from build123d import *

# Parameters (mm, degrees)
SKETCH1_R                = 103.1875
BASE_FLANGE1_DEPTH       = 4.7752
SKETCH6_R                = 4.9609375
CUT_EXTRUDE1_DEPTH       = 147.007269845
SKETCH7_R                = 38.1
CUT_EXTRUDE2_DEPTH       = 147.007269845
CUT_EXTRUDE6_DEPTH       = 147.007269845
FILLET2_R                = 1.5875
FILLET3_R                = 8.466666667
CIRPATTERN3_COUNT        = 14
FILLET2_OF_CIRPATTERN3_R = 1.5875
FILLET3_OF_CIRPATTERN3_R = 8.466666667


# Sheet-metal steps are written as plain solids
with BuildPart() as part:
    # Sketch1 → Base-Flange1 (new body)
    with BuildSketch(Plane.XY):
        Circle(SKETCH1_R)
    extrude(amount=-BASE_FLANGE1_DEPTH)

    # Sketch6 → Cut-Extrude1 (cut, through all)
    with BuildSketch(Plane.XY):
        with Locations((0, 47.534367171)):
            Circle(SKETCH6_R)
        with Locations((45.207869646, 14.688927273)):
            Circle(SKETCH6_R)
        with Locations((27.94, -38.456110858)):
            Circle(SKETCH6_R)
        with Locations((-27.94, -38.456110858)):
            Circle(SKETCH6_R)
        with Locations((-45.207869646, 14.688927273)):
            Circle(SKETCH6_R)
    extrude(amount=-CUT_EXTRUDE1_DEPTH, mode=Mode.SUBTRACT)

    # Sketch7 → Cut-Extrude2 (cut, through all)
    with BuildSketch(Plane.XY):
        Circle(SKETCH7_R)
    extrude(amount=-CUT_EXTRUDE2_DEPTH, mode=Mode.SUBTRACT)

    # Sketch14 → Cut-Extrude6 (cut, through all)
    with BuildSketch(Plane.XY):
        with BuildLine():
            ThreePointArc((0, 96.8375), (16.707624198, 79.710005113), (29.767032143, 59.661372951))
            ThreePointArc((29.767032143, 59.661372951), (25.116422432, 61.763427279), (20.318653947, 63.50360562))
            ThreePointArc((20.318653947, 63.50360562), (6.935369559, 81.376622779), (-9.620686715, 96.358413195))
            ThreePointArc((-9.620686715, 96.358413195), (-4.816304004, 96.717654138), (0, 96.8375))
        make_face()
    cut_extrude6 = extrude(amount=-CUT_EXTRUDE6_DEPTH, mode=Mode.SUBTRACT)

    # Fillet2
    fillet2_edges = [part.edges().sort_by_distance(p)[0] for p in [
        (-9.620686715, 96.358413195, -2.3876),
        (29.767032143, 59.661372951, -2.3876),
    ]]
    fillet(fillet2_edges, radius=FILLET2_R)

    # Fillet3
    fillet3_edges = [part.edges().sort_by_distance(p)[0] for p in [
        (0, 96.8375, -2.3876),
        (20.318653947, 63.50360562, -2.3876),
    ]]
    fillet(fillet3_edges, radius=FILLET3_R)

    # CirPattern3: Cut-Extrude6 ×14 about axis
    cirpattern3_axis = Axis((0, 0, 0), (0, 0, 1))
    for i in range(1, CIRPATTERN3_COUNT):
        add(cut_extrude6.rotate(cirpattern3_axis, i * 360 / CIRPATTERN3_COUNT), mode=Mode.SUBTRACT)

    # Fillet2 of CirPattern3
    fillet2_of_cirpattern3_edges = [part.edges().sort_by_distance(p)[0] for p in [
        (-50.47628783, 82.641670924, -2.3876),
        (0.933069674, 66.668470854, -2.3876),
        (-81.33444109, 52.556732194, -2.3876),
        (-28.085698687, 60.471060469, -2.3876),
        (-96.08331079, 12.062288086, -2.3876),
        (-51.541749975, 42.296614929, -2.3876),
        (-91.801702404, -30.821240111, -2.3876),
        (-64.789325562, 15.744806069, -2.3876),
        (-69.337640983, -67.600243707, -2.3876),
        (-65.204580633, -13.92545473, -2.3876),
        (-33.140409395, -90.990189973, -2.3876),
        (-52.705268828, -40.837608436, -2.3876),
        (9.620686715, -96.358413195, -2.3876),
        (-29.767032143, -59.661372951, -2.3876),
        (50.47628783, -82.641670924, -2.3876),
        (-0.933069674, -66.668470854, -2.3876),
        (81.33444109, -52.556732194, -2.3876),
        (28.085698687, -60.471060469, -2.3876),
        (96.08331079, -12.062288086, -2.3876),
        (51.541749975, -42.296614929, -2.3876),
        (91.801702404, 30.821240111, -2.3876),
        (64.789325562, -15.744806069, -2.3876),
        (69.337640983, 67.600243707, -2.3876),
        (65.204580633, 13.92545473, -2.3876),
        (33.140409395, 90.990189973, -2.3876),
        (52.705268828, 40.837608436, -2.3876),
    ]]
    fillet(fillet2_of_cirpattern3_edges, radius=FILLET2_OF_CIRPATTERN3_R)

    # Fillet3 of CirPattern3
    fillet3_of_cirpattern3_edges = [part.edges().sort_by_distance(p)[0] for p in [
        (-42.016216587, 87.247572746, -2.3876),
        (-9.24670721, 66.030705212, -2.3876),
        (-75.710606183, 60.377193687, -2.3876),
        (-36.980644601, 55.479613823, -2.3876),
        (-94.409581696, 21.548370942, -2.3876),
        (-57.39011179, 33.940104503, -2.3876),
        (-94.409581696, -21.548370942, -2.3876),
        (-66.432763496, 5.678341239, -2.3876),
        (-75.710606183, -60.377193687, -2.3876),
        (-62.317591648, -23.708087148, -2.3876),
        (-42.016216587, -87.247572746, -2.3876),
        (-45.859656498, -48.398838115, -2.3876),
        (0, -96.8375, -2.3876),
        (-20.318653947, -63.50360562, -2.3876),
        (42.016216587, -87.247572746, -2.3876),
        (9.24670721, -66.030705212, -2.3876),
        (75.710606183, -60.377193687, -2.3876),
        (36.980644601, -55.479613823, -2.3876),
        (94.409581696, -21.548370942, -2.3876),
        (57.39011179, -33.940104503, -2.3876),
        (94.409581696, 21.548370942, -2.3876),
        (66.432763496, -5.678341239, -2.3876),
        (75.710606183, 60.377193687, -2.3876),
        (62.317591648, 23.708087148, -2.3876),
        (42.016216587, 87.247572746, -2.3876),
        (45.859656498, 48.398838115, -2.3876),
    ]]
    fillet(fillet3_of_cirpattern3_edges, radius=FILLET3_OF_CIRPATTERN3_R)


solid = part.part
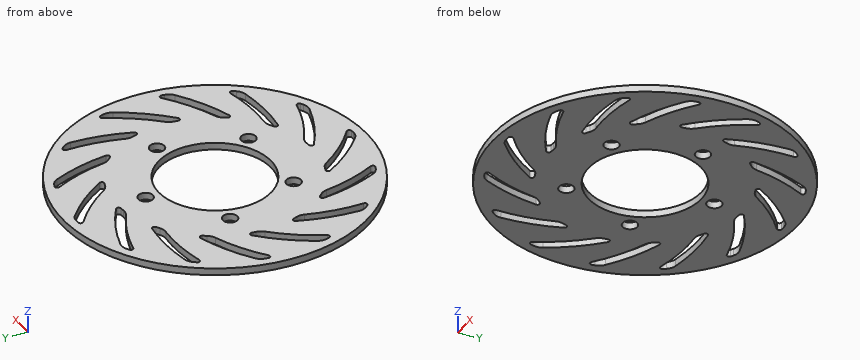
Design review of the part built by this model. Coordinates are the model's own, in mm. Coordinates: 2 decimals unless noted, no trailing zeros. Write each loop counter-clockwise with the first axis right and the second up, starting at its lowest first coordinate (ties: lowest second). Pieces come first, ordered by that corner, then holes. Notation, with made-up numbers: (-39.75, 62) - (-23.75, 62) arc R31 ccw to (-23.75, 100) - close; hole circle Ø3 at (-29.75, 7). An arc over 180 degrees is marked (long way). One line per item, written item: value.
1) To check wall thickness, follow probe 1 along Y at (x, z) = (-27.94, -2.8); probe 2 along X at (y, z) = (-71.5, -1.3); probe 3 along X at (y, z) = (-50, -3.6). State the ranges of each line that lie inside material, in increasing order.
Answer sheet:
probe 1: y = -99.33 to -43.42, -33.5 to -25.9, 25.9 to 75.87, 82.71 to 99.33
probe 2: x = -74.4 to -47.83, -41.19 to -22.74, -14.99 to 6.01, 18.61 to 74.4
probe 3: x = -90.26 to -74.99, -68.6 to -52.08, -45.8 to 90.26
2) Add section C-C (z = -2.15). Give the number of separate pieces and of enclosed holes in the cut face, plus the area to 3 significant figures.
Answer sheet:
separate pieces: 1
enclosed holes: 20
area: 24,500 mm2
3) Add section B-B (y = 0). State the section outline as (x, z) points, plus the area to 3 significant figures.
Answer sheet:
outline: (-103.19, -4.78) - (-80.26, -4.78) - (-80.26, 0) - (-103.19, 0) - close; (-71.9, -4.78) - (-38.1, -4.78) - (-38.1, 0) - (-71.9, 0) - close; (38.1, -4.78) - (71.9, -4.78) - (71.9, 0) - (38.1, 0) - close; (80.26, -4.78) - (103.19, -4.78) - (103.19, 0) - (80.26, 0) - close
area: 542 mm2
4) Add section A-A (x = 83). State the section outline as (y, z) points.
Answer sheet:
outline: (-61.31, -4.78) - (-29.19, -4.78) - (-29.19, 0) - (-61.31, 0) - close; (-21.74, -4.78) - (3.47, -4.78) - (3.47, 0) - (-21.74, 0) - close; (14.51, -4.78) - (61.31, -4.78) - (61.31, 0) - (14.51, 0) - close
5) Insertion check: pin 1 (13 mm diameter, centred on x = 0, y = 47.53, fed in from +Z); pin 2 (1 mm diameter, centred on y = 60.5, z = -2, fed in from -X). Each pin has a flat end and moves straight along its axis. Give the tip position at first contact, or say it passes through.
Answer sheet:
pin 1: stops at z = 0
pin 2: stops at x = -83.95
